```python
from build123d import *

# Parameters (mm, degrees)
ESBO_O1_R                = 4
RESSALTO_EXTRUS_O1_DEPTH = 1
ESBO_O2_R                = 2
RESSALTO_EXTRUS_O2_DEPTH = 0.5
ESBO_O3_W                = 6.92820323
ESBO_O3_H                = 4
RESSALTO_EXTRUS_O3_DEPTH = 1


with BuildPart() as part:
    # Esboço1 → Ressalto-extrusão1 (new body)
    with BuildSketch(Plane.XY):
        Circle(ESBO_O1_R)
    extrude(amount=RESSALTO_EXTRUS_O1_DEPTH)

    # Esboço2 → Ressalto-extrusão2 (add)
    with BuildSketch(Plane.XY.offset(1)):
        Circle(ESBO_O2_R)
    extrude(amount=RESSALTO_EXTRUS_O2_DEPTH)

    # Esboço3 → Ressalto-extrusão3 (add)
    with BuildSketch(Plane(origin=(0, 0, 0), x_dir=(-1, 0, 0), z_dir=(0, 0, -1))):
        Rectangle(ESBO_O3_W, ESBO_O3_H)
    extrude(amount=RESSALTO_EXTRUS_O3_DEPTH)


solid = part.part
```
For this review, take the finished solid that the model builds, in its own axes (mm). A direction names the side the tool comes from. Coordinates: 2 decimals unless noted, no trailing zeros. Order: outer loops, then holes, each group sorted by start corner. A loop starts at its lowest first (then second) coordinate and runs counter-clockwise, first axis right, second up. Notation, with made-up numbers: (-21.5, 50) - (-11.5, 50) arc R26 cw to (-11.5, 72) - close; hole circle Ø6 at (-1.5, 20.5). An arc over 180 degrees is marked (long way). Answer as a JSON object with one key per item and string values. Group by question number.
1. We need section D-D on x = 3. State the section outline as (y, z) points.
2. We need section C-C on z = 0.1. State the section outline as (x, y) points, then the cut area to 3 significant figures.
3. For probe 1 along Y at (x, z) = (1, -0.35); probe 2 along Z at (x, y) = (0, 2.25); probe 3 along Z at (x, y) = (3, 1.25), list the stretches that pass through material, from the lowest coordinate up.
4. Clearance check with flat-ended pins moving along their axes: P1, Ø1, axis at y = 1, z = 0.5, coming from the +X side; P2, Ø0.6, axis at x = -1.5, y = -3.5, coming from the -Z side; P3, Ø0.8, axis at x = 0, z = -0.5, coming from the +Y side. State where each tip first meets the part, or that it passes through.
5. We need section A-A on x = 0. State the section outline as (y, z) points.
6. For faces 1 (the flat face through (-3.464, 0, -0.5)), 2 (the cylindrical face through (-0.434, -1.952, 1.246)), 3 (the flat face through (3.464, 0, -0.5)), 4 (the flat face through (0, 2, -0.5)), list the 3-axis set-ups (+Z, -Z, +X, -X, +Y, -Y) from which the entire face can be reached by the end or side of a thin tool; tool diameter is ignored.
7. We need section B-B on y = 0. State the section outline as (x, z) points.
Final values:
{
 "1": {"outline": "(-2.65, 0) - (-2, 0) - (-2, -1) - (2, -1) - (2, 0) - (2.65, 0) - (2.65, 1) - (-2.65, 1) - close"},
 "2": {"outline": "circle Ø8 at (0, 0)", "area": "50.3 mm²"},
 "3": {"probe 1": "-2 to 2", "probe 2": "0 to 1", "probe 3": "-1 to 1"},
 "4": {"P1": "x = 3.97", "P2": "z = 0", "P3": "y = 2"},
 "5": {"outline": "(-4, 0) - (-2, 0) - (-2, -1) - (2, -1) - (2, 0) - (4, 0) - (4, 1) - (2, 1) - (2, 1.5) - (-2, 1.5) - (-2, 1) - (-4, 1) - close"},
 "6": {"face 1": "-Z, -X, +Y, -Y", "face 2": "+Z", "face 3": "-Z, +X, +Y, -Y", "face 4": "-Z, +X, -X, +Y"},
 "7": {"outline": "(-4, 0) - (-3.46, 0) - (-3.46, -1) - (3.46, -1) - (3.46, 0) - (4, 0) - (4, 1) - (2, 1) - (2, 1.5) - (-2, 1.5) - (-2, 1) - (-4, 1) - close"}
}
